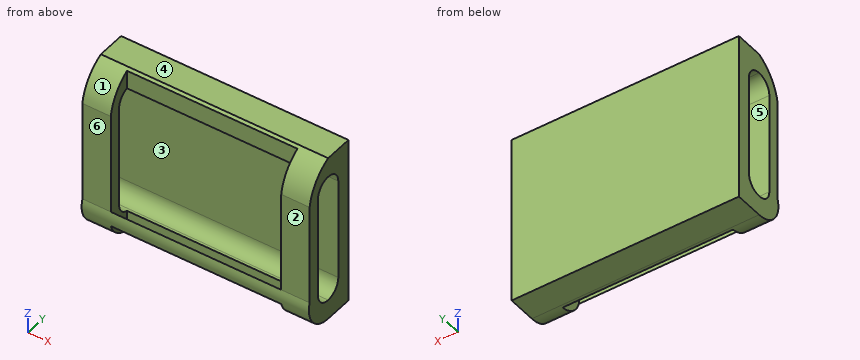
```python
from build123d import *

# Parameters (mm, degrees)
F0_W     = 50.8
F0_H     = 38.1
F1_DEPTH = 6.35
F3_DEPTH = 50.8
F5_DEPTH = 101.6
F6_W     = 38.1
F6_H     = 22.6706631617
F6_H_2   = 10.8896684192
F7_DEPTH = 5.08


with BuildPart() as f1:
    # F0 (on Front) → F1 (new body)
    with BuildSketch(Plane.XZ):
        Rectangle(F0_W, F0_H)
    extrude(amount=F1_DEPTH)

    # F2 (on face) → F3 (join)
    with BuildSketch(Plane(origin=(-25.4, 0, 0), x_dir=(0, -1, 0), z_dir=(-1, 0, 0))):
        with BuildLine():
            ThreePointArc((6.35, 14.6177), (8.6040442864, 13.6840442864), (9.5377, 11.43))
            ThreePointArc((9.5377, 11.43), (8.6040442864, 9.1759557136), (6.35, 8.2423))
            Line((6.35, 8.2423), (6.35, -8.2423))
            ThreePointArc((6.35, -8.2423), (8.6040442864, -9.1759557136), (9.5377, -11.43))
            ThreePointArc((9.5377, -11.43), (8.6040442864, -13.6840442864), (6.35, -14.6177))
            Line((6.35, -14.6177), (6.35, -19.05))
            ThreePointArc((6.35, -19.05), (11.173439943, -16.6397561834), (12.1419066563, -11.3353315808))
            Line((12.1419066563, -11.3353315808), (12.1419066563, 11.3353315808))
            ThreePointArc((12.1419066563, 11.3353315808), (10.2292171372, 15.9308663055), (6.35, 19.05))
            Line((6.35, 19.05), (6.35, 14.6177))
        make_face()
    extrude(amount=-F3_DEPTH)

    # F4 (on face) → F5 (cut)
    with BuildSketch(Plane(origin=(-25.4, 0, 0), x_dir=(0, -1, 0), z_dir=(-1, 0, 0))):
        with BuildLine():
            Line((6.35, 8.2423), (6.35, 14.6177))
            ThreePointArc((6.35, 14.6177), (4.0959557136, 13.6840442864), (3.1623, 11.43))
            ThreePointArc((3.1623, 11.43), (4.0959557136, 9.1759557136), (6.35, 8.2423))
        make_face()
        with BuildLine():
            ThreePointArc((6.35, 8.2423), (8.6040442864, 9.1759557136), (9.5377, 11.43))
            ThreePointArc((9.5377, 11.43), (8.6040442864, 13.6840442864), (6.35, 14.6177))
            Line((6.35, 14.6177), (6.35, 8.2423))
        make_face()
        with BuildLine():
            Line((6.35, -14.6177), (6.35, -8.2423))
            ThreePointArc((6.35, -8.2423), (4.0959557136, -9.1759557136), (3.1623, -11.43))
            ThreePointArc((3.1623, -11.43), (4.0959557136, -13.6840442864), (6.35, -14.6177))
        make_face()
        with BuildLine():
            ThreePointArc((6.35, -14.6177), (8.6040442864, -13.6840442864), (9.5377, -11.43))
            ThreePointArc((9.5377, -11.43), (8.6040442864, -9.1759557136), (6.35, -8.2423))
            Line((6.35, -8.2423), (6.35, -14.6177))
        make_face()
        with BuildLine():
            Line((9.5377, -11.43), (9.5377, 11.43))
            ThreePointArc((9.5377, 11.43), (8.6040442864, 9.1759557136), (6.35, 8.2423))
            ThreePointArc((6.35, 8.2423), (4.0959557136, 9.1759557136), (3.1623, 11.43))
            Line((3.1623, 11.43), (3.1623, -11.43))
            ThreePointArc((3.1623, -11.43), (4.0959557136, -9.1759557136), (6.35, -8.2423))
            ThreePointArc((6.35, -8.2423), (8.6040442864, -9.1759557136), (9.5377, -11.43))
        make_face()
    extrude(amount=-F5_DEPTH, mode=Mode.SUBTRACT)

    # F6 (on face) → F7 (cut)
    with BuildSketch(Plane.XZ.offset(12.1419066563)):
        Rectangle(F6_W, F6_H)
        with Locations((0, 16.7801657904)):
            Rectangle(F6_W, F6_H_2)
        with Locations((0, -16.7801657904)):
            Rectangle(F6_W, F6_H_2)
    extrude(amount=-F7_DEPTH, mode=Mode.SUBTRACT)


solid = f1.part
```
Can you work these out from the model? Positions are in its coordinate system, mm. Face numbers are marked on the shaded views. A direction names the side the tool comes from. Give positions to 0.01 mm unless a question says otherwise; leave off trailing zeros. Loops run counter-clockwise (first coordinate to the right, second up) from the corner with the lowest first, then second, coordinate; pieces in that order, holes last. Notation, with made-up numbers: M 46.5,82 L 104.5,82 A9 cw 104.5,94 Z; hole C 39.25,5 d8. An arc over 180 degrees is marked long. One line per item, written item: value.
(1) We'd pull the mould along Z, two halves only. Please class the marked faces 1, 2 and 3: released by +Z, released by -Z, zero draft, split by the parting line, or undercut.
Returned:
face 1: released by +Z
face 2: zero draft
face 3: undercut
(2) Suppose I cut it at B-B on x = -21.5. List the corners of the cut face in (y, z) for me, plus the area to 3 significant figures.
Returned:
outline: M -12.14,-11.34 A6.03 ccw -6.35,-19.05 L 0,-19.05 L 0,19.05 L -6.35,19.05 A10.08 ccw -12.14,11.34 Z; hole M -9.54,-11.43 A3.19 ccw -3.16,-11.43 L -3.16,11.43 A3.19 ccw -9.54,11.43 Z
area: 265 mm^2
(3) Suppose I cut it at C-C on x = -12.5. List the corners of the cut face in (y, z) for me, plus the area to 3 significant figures.
Returned:
outline: M -12.14,-14.7 L -12.14,-11.34 A6.03 ccw Z; M -7.06,-19.01 A6.03 ccw -6.35,-19.05 L 0,-19.05 L 0,19.05 L -6.35,19.05 A10.08 ccw -7.06,18.69 L -7.06,14.54 A3.19 cw -3.16,11.43 L -3.16,-11.43 A3.19 cw -7.06,-14.54 Z
area: 160 mm^2
(4) I need wall thicknesses on line 1 (Y direction, x = -21, z = 5); line 2 (X direction, y = -11.25, z = 11); line 3 (Y direction, x = -8.5, z = 16.5). Which ranges of each line are inside material? Lowest first, please.
Returned:
line 1: -12.14 to -9.54, -3.16 to 0
line 2: -25.4 to -19.05, 19.05 to 25.4
line 3: -7.06 to 0
(5) Suppose I cut it at D-D on y = -4.5. List the corners of the cut face in (x, z) for me, plus the area to 3 significant figures.
Returned:
outline: M -25.4,-19.05 L 25.4,-19.05 L 25.4,-14.03 L -25.4,-14.03 Z; M -25.4,14.03 L 25.4,14.03 L 25.4,19.05 L -25.4,19.05 Z
area: 510 mm^2
(6) Suppose I cut it at A-A on z = 1. List the corners of the cut face in (x, y) for me.
Returned:
outline: M -25.4,-12.14 L -19.05,-12.14 L -19.05,-9.54 L -25.4,-9.54 Z; M -25.4,-3.16 L 25.4,-3.16 L 25.4,0 L -25.4,0 Z; M 19.05,-12.14 L 25.4,-12.14 L 25.4,-9.54 L 19.05,-9.54 Z
(7) Which directions (+Z, -Z, +X, -X, +Y, -Y) give clear straight access to the entire face, cutting with the end or side of a thin tool? Please do the marked faces 4, 5 and 6.
Returned:
face 4: +Z, +X, -X, +Y, -Y
face 5: +X, -X
face 6: +Z, +X, -X, -Y
(8) Will these pins go through, and if not, where does the flat tip stop? pin 1 (1 mm diameter, centred on x = 12, y = -7.5, fed in from +Z); pin 2 (7 mm diameter, centred on x = 21.5, z = -0.5, fed in from -Y); pin 3 (3 mm diameter, centred on x = -22.5, z = -0.5, fed in from +Y); pin 4 (2 mm diameter, centred on x = -16, z = 14, fed in from -Y).
Returned:
pin 1: z = 18.72
pin 2: y = -12.14
pin 3: y = 0
pin 4: y = -7.06
